Check sheet for the drawn part. Datum: minimum x, y, z corner. Units: mm. Round coordinates to 2 decimals unless told otherwise and drop trailing zeros. Write each loop counter-clockwise with the first axis right and the second up, starting at its lowest first coordinate (ties: lowest second). Pieces come first, ordered by that corner, then holes.
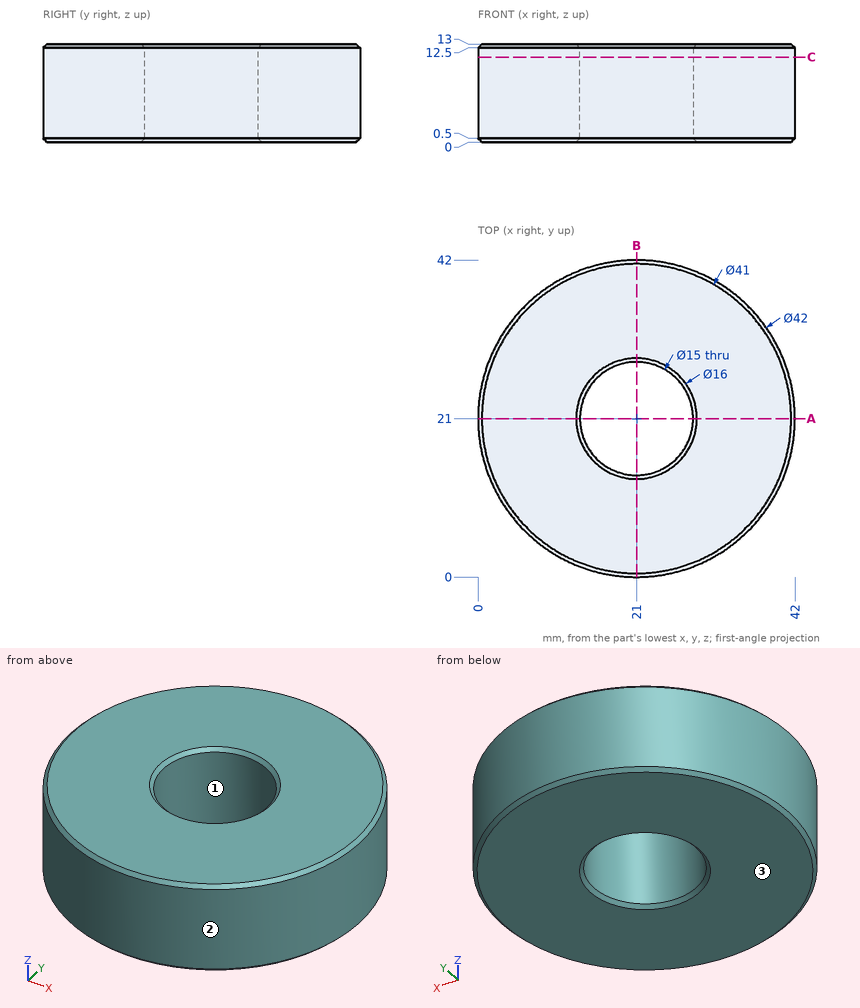
1. Scan lines: line 1 along Y through (x, z) = (21, 3.5); line 2 along Y through (x, z) = (22, 4); line 3 along X through (y, z) = (27.5, 3). Record each from-to range of solid material in increasing order.
2. Sectioned sample at C-C, the plane z = 11.25. Enter the section's corners in (x, y).
3. Release check for a two-part mould opening along Y. For the marked faces 1, 2 and 3 record: released by +Y, released by -Y, zero draft, split by the parting line, or undercut.
4. Go/stop test with flat-tipped pins: pin 1 (3 mm diameter, centred on x = 17, z = 8, fed in from -Y); pin 2 (5 mm diameter, centred on x = 14.5, z = 7, fed in from +Y); pin 3 (3 mm diameter, centred on x = 25.5, z = 1.5, fed in from +Y); pin 4 (12 mm diameter, centred on x = 21, y = 21, fed in from +Z). Record where each tip stops, or that it passes through.
5. Sectioned sample at A-A, the plane y = 21. Enter the section's corners in (x, z).
Computed values:
1. line 1: y = 0 to 13.5, 28.5 to 42
1. line 2: y = 0.02 to 13.57, 28.43 to 41.98
1. line 3: x = 1.03 to 17.26, 24.74 to 40.97
2. outline: circle Ø42 at (21, 21); hole circle Ø15 at (21, 21)
3. face 1: undercut
3. face 2: split by the parting line
3. face 3: zero draft
4. pin 1: stops at y = 0.15
4. pin 2: stops at y = 41.62
4. pin 3: stops at y = 41.78
4. pin 4: passes through
5. outline: (0, 0.5) - (0.5, 0) - (13, 0) - (13.5, 0.5) - (13.5, 12.5) - (13, 13) - (0.5, 13) - (0, 12.5) - close; (28.5, 0.5) - (29, 0) - (41.5, 0) - (42, 0.5) - (42, 12.5) - (41.5, 13) - (29, 13) - (28.5, 12.5) - close
